Autodesk Inventor part; units mm, degrees
ref_plane "YZ Plane" through (0, 0, 0) normal (1, 0, 0) x (0, 1, 0)
ref_plane "XZ Plane" through (0, 0, 0) normal (0, 1, 0) x (-1, 0, 0)
ref_plane "XY Plane" through (0, 0, 0) normal (0, 0, 1) x (1, 0, 0)
sketch "Sketch4" plane through (0, 0, 0) normal (0, 0, 1) x (1, 0, 0)
  line L0 (-10, -18) -> (10, -18)
  line L1 (10, -18) -> (10, 18)
  line L2 (10, 18) -> (-10, 18)
  line L3 (-10, 18) -> (-10, -18)
  line L4 (-10, -18) -> (10, 18) construction
  line L5 (10, -18) -> (-10, 18) construction
  point P0 (0, 0)
  dimension "d16" = 20
  dimension "d17" = 36
extrude "Extrusion4" add sketch "Sketch4" along normal blind 2
sketch "Sketch5" plane through (0, 0, 2) normal (0, 0, 1) x (1, 0, 0)
  line L0 (0, 25.2) -> (0, -25.2)
  circle A0 centre (0, 13) radius 2.25
  circle A1 centre (0, -13) radius 2.25
  line L1 (10, 18) -> (-10, 18)
  line L2 (-10, -18) -> (10, -18)
  point P0 (0, 0)
  dimension "d20" = 4.5
  dimension "d21" = 4.5
  dimension "d22" = 5
  dimension "d23" = 5
extrude "Extrusion5" cut sketch "Sketch5" against normal through all
sketch "Sketch6" plane through (0, 0, 2) normal (0, 0, 1) x (1, 0, 0)
  circle A0 centre (0, 0) radius 8
  dimension "d26" = 16
extrude "Extrusion6" add sketch "Sketch6" along normal blind 2
fillet "Fillet1" radius 2 4 edges at (10, 18, 1) (-10, 18, 1) (-10, -18, 1) (10, -18, 1)
sketch "Sketch7" plane through (0, 0, 4) normal (0, 0, 1) x (1, 0, 0)
  circle A0 centre (0, 0) radius 3.5
  dimension "d30" = 7
extrude "Extrusion7" add sketch "Sketch7" along normal blind 6
chamfer "Chamfer1" distance 2 angle 45 1 edges at (-3.5, 0, 4)
sketch "Sketch8" plane through (0, 0, 10) normal (0, 0, 1) x (1, 0, 0)
  circle A0 centre (0, 0) radius 2.25
  dimension "d36" = 4.5
extrude "Extrusion8" cut sketch "Sketch8" against normal through all
chamfer "Chamfer2" distance 3 angle 45 1 edges at (-2.25, 0, 0)
sketch "Sketch10" plane through (0, 0, 10) normal (0, 0, 1) x (1, 0, 0)
  circle A0 centre (0, 0) radius 13.6126
extrude "Extrusion9" cut sketch "Sketch10" against normal blind 5
equation "\"d21\" = d20"
equation "\"d23\" = d22"
properties part number "LinearActuatorHolder"
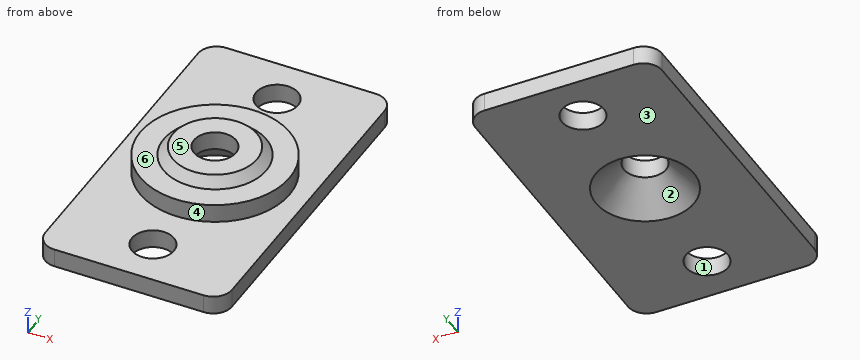
Part model, mm, in its own coordinate system. Face numbers are marked on the shaded views. A direction names the side the tool comes from. Give positions to 0.01 mm unless a question says otherwise; leave off trailing zeros. Order: outer loops, then holes, each group sorted by start corner. A loop starts at its lowest first (then second) coordinate and runs counter-clockwise, first axis right, second up. Notation, with made-up numbers: (-9.5, -28.5) - (44.5, -28.5) arc R13 cw to (44.5, -20.5) - close; hole circle Ø3 at (67.25, 84). An arc over 180 degrees is marked (long way). Use a Markdown table: item, result.
1) 3-axis set-ups, long thin cutter, end or side, ignore diameter. For the marked faces 5 and 6: which of +Z, -Z, +X, -X, +Y, -Y reach the whole face in a straight line?
Checked values:
| item | result |
|---|---|
| face 5 | +Z, +X, -X, +Y, -Y |
| face 6 | +Z |
2) Saw through at A-A on y = 0. List the corners of the cut face in (x, z), plus the area to 3 significant figures.
Checked values:
| item | result |
|---|---|
| outline | (-10, 0) - (-5.25, 0) - (-2.25, 3) - (-2.25, 5) - (-4.5, 5) - (-5.5, 4) - (-8, 4) - (-8, 2) - (-10, 2) - close; (2.25, 3) - (5.25, 0) - (10, 0) - (10, 2) - (8, 2) - (8, 4) - (5.5, 4) - (4.5, 5) - (2.25, 5) - close |
| area | 50.5 mm² |
3) Saw through at B-B on z = 0.9. List the corners of the cut face in (x, y), plus the area to 3 significant figures.
Checked values:
| item | result |
|---|---|
| outline | (-10, -16) arc R2 ccw to (-8, -18) - (8, -18) arc R2 ccw to (10, -16) - (10, 16) arc R2 ccw to (8, 18) - (-8, 18) arc R2 ccw to (-10, 16) - close; hole circle Ø8.7 at (0, 0); hole circle Ø4.5 at (0, -13); hole circle Ø4.5 at (0, 13) |
| area | 625 mm² |
4) Saw through at D-D on z = 2.65. List the corners of the cut face in (x, y).
Checked values:
| item | result |
|---|---|
| outline | circle Ø16 at (0, 0); hole circle Ø5.2 at (0, 0) |
5) Probe L1, parallel to Y at x = -1, z = 0.95; L2, parallel to X at y = 13, z = 0.65; L3, parallel to Y at x = 0, z = 0.65. List the from-to ranges inside material, lowest first. Write a range as from..to.
Checked values:
| item | result |
|---|---|
| L1 | -18..-15.02, -10.98..-4.18, 4.18..10.98, 15.02..18 |
| L2 | -10..-2.25, 2.25..10 |
| L3 | -18..-15.25, -10.75..-4.6, 4.6..10.75, 15.25..18 |
6) Flat gauge pins, fed straight in: P1, Ø1, axis at y = 3, z = 3, coming from the +X side; P2, Ø5, axis at x = 0, y = 0, coming from the -Z side. Where does each tip first touch, or does it go through?
Checked values:
| item | result |
|---|---|
| P1 | x = 7.6 |
| P2 | z = 2.75 |
7) Saw through at C-C on x = 0. List the corners of the cut face in (y, z), plus the area to 3 significant figures.
Checked values:
| item | result |
|---|---|
| outline | (-18, 0) - (-15.25, 0) - (-15.25, 2) - (-18, 2) - close; (-10.75, 0) - (-5.25, 0) - (-2.25, 3) - (-2.25, 5) - (-4.5, 5) - (-5.5, 4) - (-8, 4) - (-8, 2) - (-10.75, 2) - close; (2.25, 3) - (5.25, 0) - (10.75, 0) - (10.75, 2) - (8, 2) - (8, 4) - (5.5, 4) - (4.5, 5) - (2.25, 5) - close; (15.25, 0) - (18, 0) - (18, 2) - (15.25, 2) - close |
| area | 64.5 mm² |
8) Two-plate mould, pull along X, no slides. Class the marked faces 1, 2, 3 and 4: +X half, -X half, draft (parallel to the pull), parting line (faces both ways), or undercut.
Checked values:
| item | result |
|---|---|
| face 1 | undercut |
| face 2 | undercut |
| face 3 | draft |
| face 4 | parting line |
